Autodesk Inventor part; units mm, degrees
ref_plane "YZ Plane" through (0, 0, 0) normal (1, 0, 0) x (0, 1, 0)
ref_plane "XZ Plane" through (0, 0, 0) normal (0, 1, 0) x (-1, 0, 0)
ref_plane "XY Plane" through (0, 0, 0) normal (0, 0, 1) x (1, 0, 0)
sketch "Sketch1" plane through (0, 0, 0) normal (0, 0, 1) x (1, 0, 0)
  line L0 (-150, -86.6025) -> (0, 173.2051) construction
  line L1 (0, 173.2051) -> (150, -86.6025) construction
  line L2 (150, -86.6025) -> (-150, -86.6025) construction
  arc A0 (120.0417, -34.617) -> (30.0416, 121.2676) centre (-150, -86.6025) ccw
  arc A1 (-90, -86.6506) -> (-120.0417, -34.617) centre (-150, -86.6025) ccw
  arc A2 (120.0417, -34.617) -> (90, -86.6506) centre (150, -86.6025) ccw
  arc A3 (-30.0416, 121.2676) -> (30.0416, 121.2676) centre (0, 173.2051) ccw
  arc A4 (-30.0416, 121.2676) -> (-120.0417, -34.617) centre (150, -86.6025) ccw
  arc A5 (-90, -86.6506) -> (90, -86.6506) centre (0, 173.2051) ccw
  point P0 (0, 0)
  point P1 (0, 0)
  dimension "d0" = 300
  dimension "d2" = 120
  dimension "d3" = 275
extrude "Extrusion1" add sketch "Sketch1" along normal blind 260
sketch "Sketch2" plane through (0, 0, 0) normal (1, 0, 0) x (0, 1, 0)
  line L0 (113.2051, 260) -> (113.2051, 0)
  line L1 (113.2051, 0) -> (-101.7949, 0)
  line L2 (-101.7949, 0) -> (-101.7949, 260)
  line L3 (-101.7949, 260) -> (113.2051, 260)
  line L4 (0, 0) -> (0, 260)
  arc A0 (173.2051, 619.634) -> (173.2051, 248.8241) centre (98.2051, 434.2291) ccw
  line L5 (113.2051, 260) -> (121.2676, 260)
  line L6 (173.2051, -124.8458) -> (173.2051, 749.0749)
  line L7 (173.2051, 619.634) -> (173.2051, 248.8241)
  dimension "d6" = 75
  dimension "d7" = 400
revolve "Revolution1" cut sketch "Sketch2" angle 360 about axis through (0, 173.2051, 0) along (0, 0, 1) contours L3 A0 L6 L0 | L0 A0 L3
pattern_circular "Circular Pattern1" count 3 over 360 about axis through (0, 0, -10) along (0, 0, 1) of "Revolution1"
properties part number "VOLUME"
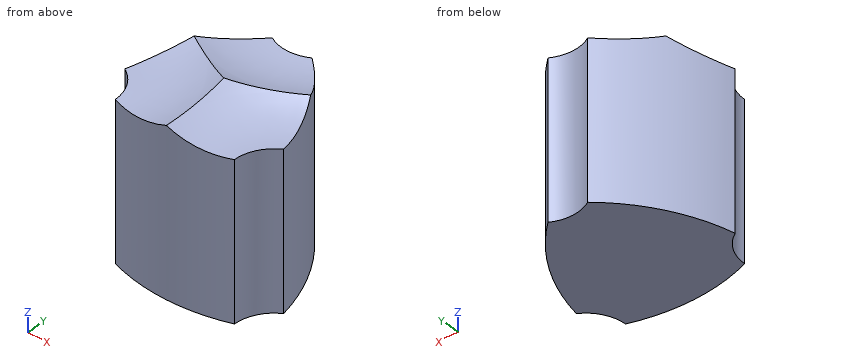
For this review, take the finished solid that the model builds, in its own axes (mm). Coordinates: 2 decimals unless noted, no trailing zeros. Write each loop counter-clockwise with the first axis right and the second up, starting at its lowest first coordinate (ties: lowest second). Pieces come first, ordered by that corner, then holes.
(1) Add section A-A on z = 82. Give the boundary of the cut face in (x, y), then the cut area to 3 significant figures.
(2) Wall thickness on probe 1 along Z at (x, y) = (98, -30.5); probe 2 along Y at (x, z) = (-52, 55.5); probe 3 along Y at (x, z) = (1.5, 140): over which ranges is each line inside the solid? List them lowest first.
(3) For pin 1 Ø1 at (x, z) = (85.5, 84) entering from +Y; pin 2 Ø4 at (y, z) = (11, 76) entering from -X; pin 3 Ø4 at (y, z) = (5, 196) entering from +X, all flat-tipped, find the tip position at first contact; note any pin that passes through.
Answer sheet:
1. outline: (-120.04, -34.62) arc R60 cw to (-90, -86.65) arc R275 ccw to (90, -86.65) arc R60 cw to (120.04, -34.62) arc R275 ccw to (30.04, 121.27) arc R60 cw to (-30.04, 121.27) arc R275 ccw to start
1. area: 38,800 mm2
2. probe 1: z = 0 to 234.23
2. probe 2: y = -96.83 to 100
2. probe 3: y = -101.79 to 113.22
3. pin 1: stops at y = 56.23
3. pin 2: stops at x = -107.85
3. pin 3: stops at x = 109.99
